Answer from the drawing. Dimensions are ordinates in mm from the lowest x, y and z of the part. A direction names the side the tool comes from. Coordinates: 2 decimals unless noted, no trailing zeros. Write each loop counter-clockwise with the first axis right and the second up, starting at its lowest first coordinate (ties: lowest second). Pieces come first, ordered by that corner, then holes.
(1) Straight lines are drawn through the part: line 1 (X direction, y = 4.35, z = 14.2); line 2 (Z direction, x = 14.2, y = 4.05); line 3 (Y direction, x = 22, z = 17.25). For each, find the intervals that lie inside material, in ascending order.
(2) For a pull along Z with two mould halves and no side action, classify the marked faces 4, 5 and 6 as +Z half, -Z half, draft (parallel to the pull), parting line (faces both ways), or undercut.
(3) The part is cut by section B-B on y = 14.5. Determine the outline of the cut face in (x, z).
(4) Given P1, Ø5, axis at x = 4.7, z = 14.2, coming from the -Y side; P2, Ø2.5, axis at x = 23.7, z = 14.2, coming from the -Y side; P3, Ø1, axis at x = 19, y = 16.5, coming from the -Z side; P4, Ø2, axis at x = 11, z = 17.5, coming from the -Y side, each flat-ended and moving along its own axis, determine where each tip first touches the part or whether it passes through.
(5) Which of the six approach directions +Z, -Z, +X, -X, +Y, -Y give full straight-line access (tool end or side, diameter ignored) to the marked faces 1, 2 and 3?
(6) The part is cut by section A-A on y = 2.5. Determine the outline of the cut face in (x, z).
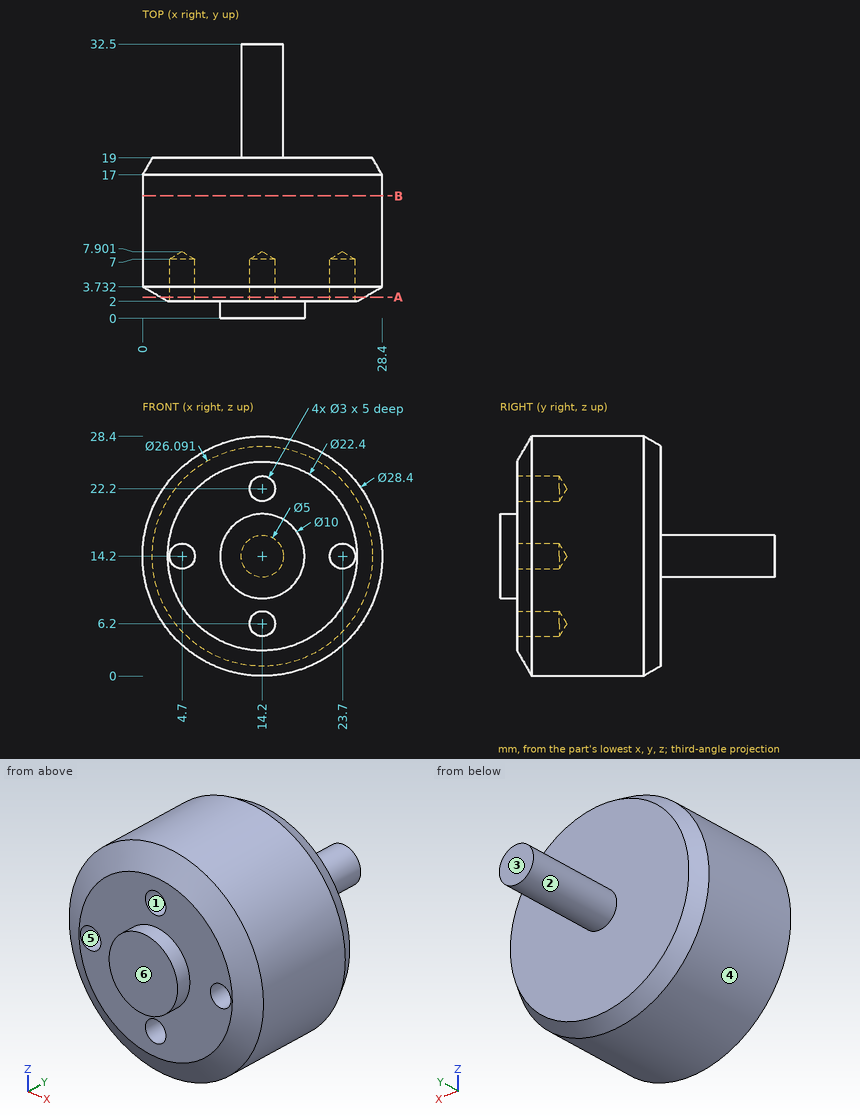
Model answer:
1. line 1: x = 0 to 3.2, 6.2 to 22.2, 25.2 to 28.4
1. line 2: z = 0 to 4.7, 7.7 to 20.7, 23.7 to 28.4
1. line 3: y = 2 to 19
2. face 4: parting line
2. face 5: undercut
2. face 6: draft
3. outline: circle Ø28.4 at (14.2, 14.2)
4. P1: stops at y = 2
4. P2: stops at y = 7.15
4. P3: stops at z = 0.67
4. P4: stops at y = 0
5. face 1: -Y
5. face 2: +Y
5. face 3: +Z, -Z, +X, -X, +Y
6. outline: circle Ø24.13 at (14.2, 14.2); hole circle Ø3 at (4.7, 14.2); hole circle Ø3 at (14.2, 6.2); hole circle Ø3 at (14.2, 22.2); hole circle Ø3 at (23.7, 14.2)
